Verification items for the finished model (mm, model axes). A direction names the side the tool comes from. Coordinates: 2 decimals unless noted, no trailing zeros. Order: outer loops, then holes, each group sorted by start corner. A loop starts at its lowest first (then second) coordinate and runs counter-clockwise, first axis right, second up. Notation, with made-up numbers: M -11.5,28.25 L 24.5,28.25 A32 cw 24.5,56.25 Z; hole C 24,48.5 d5. An arc over 180 degrees is marked long. Answer as a JSON object with one key per item and string values. Group by question number.
(1) Cross-section at D-D (y = -3.75). Enter the section's corners in (x, z), plus the area to 3 significant figures.
(2) Access from +Z, -Z, +X, -X, +Y, -Y to the whole of each face (thin tool, end or side, straight path). Record for faces 1 (the face through (30, 0, 12)), 2 (the face through (33, 0, 8)), 3 (the face through (-38.1, 0.2, 17)).
(3) Material ranges on line 1 (X direction, y = 3, z = 8.75); line 2 (Z direction, x = 35.5, y = -7.5); line 3 (X direction, y = 1.25, z = 2.5), recorded low to high.
(4) Mould release check, pull along X, two halves, no side actions. Record for faces 4 (the face through (40, 0, 20)), 5 (the face through (-33, 0, 8)), 6 (the face through (-35.21, -0.91, 19.46)), 7 (the face through (0, 12.5, 2)): released by +X, released by -X, zero draft, split by the parting line, or undercut.
(5) Cross-section at B-B (y = 0). Enter the section's corners in (x, z).
(6) Cross-section at C-C (z = 14). Enter the section's corners in (x, y).
(7) Cross-section at A-A (z = 18). Enter the section's corners in (x, y), plus the area to 3 significant figures.
(8) Gauge pin test, flat ends, axial feed: pin 1 Ø3 at (y, z) = (-5.5, 13) entering from -X; pin 2 Ø8 at (y, z) = (-5.5, 4.5) entering from +X; pin 3 Ø8 at (x, z) = (-24, 16.5) entering from -Y; pin 4 Ø5.5 at (x, y) = (-36, 1) entering from -Z. Record the tip position at first contact, or that the pin passes through.
Autodesk Inventor part; units mm, degrees
ref_plane "YZ Plane" through (0, 0, 0) normal (1, 0, 0) x (0, 1, 0)
ref_plane "XZ Plane" through (0, 0, 0) normal (0, 1, 0) x (-1, 0, 0)
ref_plane "XY Plane" through (0, 0, 0) normal (0, 0, 1) x (1, 0, 0)
sketch "Эскиз1" plane through (0, 0, 0) normal (0, 0, 1) x (1, 0, 0)
  line L0 (-30, -12.5) -> (30, -12.5)
  line L1 (30, -12.5) -> (30, 12.5)
  line L2 (30, 12.5) -> (-30, 12.5)
  line L3 (-30, 12.5) -> (-30, -12.5)
  line L4 (-30, -12.5) -> (30, 12.5) construction
  line L5 (30, -12.5) -> (-30, 12.5) construction
  point P0 (0, 0)
  dimension "d0" = 60
  dimension "d14" = 25
extrude "Выдавливание1" add sketch "Эскиз1" along normal blind 3
sketch "Эскиз2" plane through (0, 0, 3) normal (0, 0, 1) x (1, 0, 0)
  line L0 (-30, 12.5) -> (-30, -12.5)
  line L1 (-30, 12.5) -> (-33, 12.5)
  line L2 (-33, 12.5) -> (-33, -12.5)
  line L3 (-33, -12.5) -> (-30, -12.5)
  line L4 (-30, -12.5) -> (-30, 12.5)
  point P0 (0, 0)
  dimension "d3" = 3
extrude "Выдавливание2" add sketch "Эскиз2" along normal blind 19 and the other way blind 3
sketch "Эскиз3" plane through (0, 0, 22) normal (0, 0, 1) x (1, 0, 0)
  line L0 (-30, -12.5) -> (-30, 12.5)
  line L1 (-30, 12.5) -> (-40, 12.5)
  line L2 (-40, 12.5) -> (-40, -12.5)
  line L3 (-40, -12.5) -> (-30, -12.5)
  line L4 (-30, -12.5) -> (-30, 12.5)
  point P0 (0, 0)
  dimension "d8" = 10
extrude "Выдавливание3" add sketch "Эскиз3" against normal blind 5
sketch "Эскиз4" plane through (0, 0, 17) normal (0, 0, -1) x (-1, 0, 0)
  circle A0 centre (36.404, 0) radius 1.5
  line L0 (40, -12.5) -> (40, 12.5)
  point P0 (0, 0)
  point P1 (40, 0)
  dimension "d11" = 3
extrude "Выдавливание4" cut sketch "Эскиз4" against normal blind 5
mirror "Зеркальное отражение1" about plane through (0, 0, 0) normal (1, 0, 0) of "Выдавливание2", "Выдавливание3", "Выдавливание4"
properties part number "000.001.013 - Скобе прижима турбины"
Taken from the geometry:
{
 "1": {"outline": "M -40,17 L -33,17 L -33,0 L 33,0 L 33,17 L 40,17 L 40,22 L 30,22 L 30,3 L -30,3 L -30,22 L -40,22 Z", "area": "382 mm²"},
 "2": {"face 1": "+Z, +Y, -Y", "face 2": "-Z, +X, +Y, -Y", "face 3": "-Z, -X, +Y, -Y"},
 "3": {"line 1": "x = -33 to -30, 30 to 33", "line 2": "z = 17 to 22", "line 3": "x = -33 to 33"},
 "4": {"face 4": "released by +X", "face 5": "released by -X", "face 6": "undercut", "face 7": "zero draft"},
 "5": {"outline": "M -40,17 L -37.9,17 L -37.9,22 L -40,22 Z; M -34.9,17 L -33,17 L -33,0 L 33,0 L 33,17 L 34.9,17 L 34.9,22 L 30,22 L 30,3 L -30,3 L -30,22 L -34.9,22 Z; M 37.9,17 L 40,17 L 40,22 L 37.9,22 Z"},
 "6": {"outline": "M -33,-12.5 L -30,-12.5 L -30,12.5 L -33,12.5 Z; M 30,-12.5 L 33,-12.5 L 33,12.5 L 30,12.5 Z"},
 "7": {"outline": "M -40,-12.5 L -30,-12.5 L -30,12.5 L -40,12.5 Z; M 30,-12.5 L 40,-12.5 L 40,12.5 L 30,12.5 Z; hole C -36.4,0 d3; hole C 36.4,0 d3", "area": "486 mm²"},
 "8": {"pin 1": "stops at x = -33", "pin 2": "stops at x = 33", "pin 3": "passes through", "pin 4": "stops at z = 17"}
}
